Input: part model. Units: mm. Frame: model coordinates. Round coordinates to 2 decimals unless told otherwise and drop trailing zeros. Loops run counter-clockwise (first coordinate to the right, second up) from the corner with the lowest first, then second, coordinate; pieces in that order, holes last.
(1) Cut plane A-A, the plane y = 22.5. Output: boundary loops of the cut face in (x, z), and give its area (3 significant figures).
(2) Line query: line 1 (Y direction, x = 0, z = 0.85); line 2 (Y direction, x = -1, z = 1.15); line 3 (Z direction, x = -11, y = 2). Output: solid intervals per line, ascending.
(3) Cut plane D-D, the plane y = 0. Give the number of separate pieces and of enclosed holes in the cut face, and give its area (3 significant figures).
(4) Cut plane B-B, the plane z = 0.75. Output: boundary loops of the cut face in (x, y).
(5) Cut plane C-C, the plane x = 0. Output: boundary loops of the cut face in (y, z).
(6) First-contact query: pin 1 Ø3.5 at (x, y) = (-14, 0) entering from -Z. Flat tip, straight axial feed; report the tip coordinate or a pass-through.
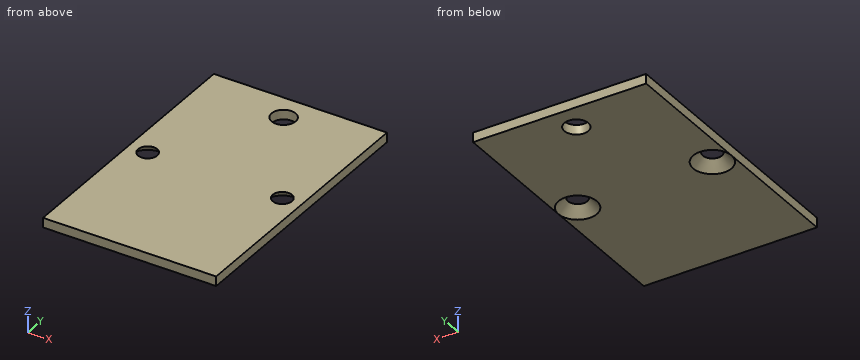
from build123d import *

# Parameters (mm, degrees)
SKETCH_W        = 36
SKETCH_H        = 56
PAD_DEPTH       = 2
SKETCH001_R     = 2
POCKET_DEPTH    = 3
CHAMFER_SIZE    = 1.99
SKETCH002_R     = 2.5
POCKET001_DEPTH = 3


with BuildPart() as part:
    # Sketch → Pad (new body)
    with BuildSketch(Plane.XY):
        Rectangle(SKETCH_W, SKETCH_H)
    extrude(amount=PAD_DEPTH)

    # Sketch001 (on Face5 of Pad) → Pocket (cut)
    with BuildSketch(Plane(origin=(0, 0, 0), x_dir=(1, 0, 0), z_dir=(0, 0, -1))):
        with Locations((14, 0)):
            Circle(SKETCH001_R)
        with Locations((-14, 0)):
            Circle(SKETCH001_R)
    extrude(amount=-POCKET_DEPTH, mode=Mode.SUBTRACT)

    # Chamfer
    chamfer_edges = [part.edges().sort_by_distance(p)[0] for p in [
        (-16, 0, 0),
        (12, 0, 0),
    ]]
    chamfer(chamfer_edges, length=CHAMFER_SIZE)

    # Sketch002 (on Face1 of Chamfer) → Pocket001 (cut)
    with BuildSketch(Plane(origin=(0, 0, 0), x_dir=(1, 0, 0), z_dir=(0, 0, -1))):
        with Locations((0, -22.5)):
            Circle(SKETCH002_R)
    extrude(amount=-POCKET001_DEPTH, mode=Mode.SUBTRACT)


solid = part.part
Reported:
1. outline: (-18, 0) - (-2.5, 0) - (-2.5, 2) - (-18, 2) - close; (2.5, 0) - (18, 0) - (18, 2) - (2.5, 2) - close
1. area: 62.0 mm2
2. line 1: y = -28 to 20, 25 to 28
2. line 2: y = -28 to 20.21, 24.79 to 28
2. line 3: z = 0.38 to 2
3. separate pieces: 3
3. enclosed holes: 0
3. area: 48.1 mm2
4. outline: (-18, -28) - (18, -28) - (18, 28) - (-18, 28) - close; hole circle Ø6.48 at (-14, 0); hole circle Ø5 at (0, 22.5); hole circle Ø6.48 at (14, 0)
5. outline: (-28, 0) - (20, 0) - (20, 2) - (-28, 2) - close; (25, 0) - (28, 0) - (28, 2) - (25, 2) - close
6. pin 1: passes through
